```python
from build123d import *

# Parameters (mm, degrees)
EXTRUDE_448_DEPTH     = 2
SKETCH_2_R            = 2
CUT_EXTRUDE_659_DEPTH = 83.412799184
SKETCH_3_R            = 2
CUT_EXTRUDE_885_DEPTH = 83.412799184


with BuildPart() as part:
    # Эскиз1 → Extrude 448 (new body)
    with BuildSketch(Plane(origin=(0, 0, 0), x_dir=(1, 0, 0), z_dir=(0, 1, 0))):
        with BuildLine():
            Line((-77.703225806, 4.495408688), (-0.361290323, 7.991837667))
            Line((-0.361290323, 7.991837667), (0.361290323, 7.991837667))
            Line((0.361290323, 7.991837667), (77.703225806, 4.495408688))
            ThreePointArc((77.703225806, 4.495408688), (82, 0), (77.703225806, -4.495408688))
            Line((77.703225806, -4.495408688), (0.361290323, -7.991837667))
            Line((0.361290323, -7.991837667), (-0.361290323, -7.991837667))
            Line((-0.361290323, -7.991837667), (-77.703225806, -4.495408688))
            ThreePointArc((-77.703225806, -4.495408688), (-82, 0), (-77.703225806, 4.495408688))
        make_face()
    extrude(amount=EXTRUDE_448_DEPTH)

    # Эскиз2 → Cut-Extrude 659 (cut, through all)
    with BuildSketch(Plane(origin=(0, 2, 0), x_dir=(1, 0, 0), z_dir=(0, 1, 0))):
        with Locations(Location((0, 0, 0), (0, 0, 270))):
            Circle(SKETCH_2_R)
    extrude(amount=-CUT_EXTRUDE_659_DEPTH, mode=Mode.SUBTRACT)

    # Эскиз3 → Cut-Extrude 885 (cut, through all)
    with BuildSketch(Plane(origin=(0, 2, 0), x_dir=(1, 0, 0), z_dir=(0, 1, 0))):
        with Locations(Location((-77.5, 0, 0), (0, 0, 270))):
            Circle(SKETCH_3_R)
        with Locations(Location((77.5, 0, 0), (0, 0, 270))):
            Circle(SKETCH_3_R)
    extrude(amount=-CUT_EXTRUDE_885_DEPTH, mode=Mode.SUBTRACT)


solid = part.part
```
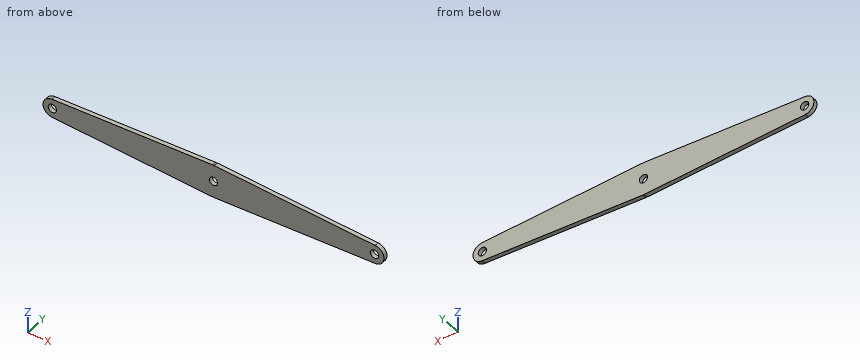
CAD build for the part. Positions are in the model's coordinates, mm. Round coordinates to 2 decimals unless told otherwise and drop trailing zeros. Write each loop counter-clockwise with the first axis right and the second up, starting at its lowest first coordinate (ties: lowest second). Pieces come first, ordered by that corner, then holes. Notation, with made-up numbers: (-18.75, -3.75) - (26.25, -3.75) arc R29 cw to (26.25, 27.25) - close; hole circle Ø4 at (77.5, 44). An arc over 180 degrees is marked (long way). Write item = value, one per line. Start each with the question number.
Q1. Band-saw the part on C-C (x = -35.5). Give the cut face in (y, z), then the cut area to 3 significant figures.
Q2. Band-saw the part on B-B (y = 1.15). Give the cut face in (x, z), then the cut area to 3 significant figures.
Q3. Band-saw the part on A-A (z = 0). Give the cut face in (x, y).
Q4. Drop a flat-ended pin along its axis: pin 1 (1.5 mm diameter, centred on x = -58.5, z = 6.5, fed in from -Y). Give the stop position or say it passes through.
Q5. Band-saw the part on D-D (x = 20.5). Give the cut face in (y, z).
Q6. Probe L1, parallel to Z at x = 37, y = 1.4; L2, parallel to Z at x = 66.5, y = 0.65. List the from-to ranges inside material, lowest first. Write a range as from..to.
Answers below:
q1.outline = (0, -6.4) - (2, -6.4) - (2, 6.4) - (0, 6.4) - close
q1.area = 25.6 mm2
q2.outline = (-77.7, -4.5) - (-0.36, -7.99) - (0.36, -7.99) - (77.7, -4.5) arc R4.5 ccw to (77.7, 4.5) - (0.36, 7.99) - (-0.36, 7.99) - (-77.7, 4.5) arc R4.5 ccw to start; hole circle Ø4 at (-77.5, 0); hole circle Ø4 at (0, 0); hole circle Ø4 at (77.5, 0)
q2.area = 1,970 mm2
q3.outline = (-82, 0) - (-79.5, 0) - (-79.5, 2) - (-82, 2) - close; (-75.5, 0) - (-2, 0) - (-2, 2) - (-75.5, 2) - close; (2, 0) - (75.5, 0) - (75.5, 2) - (2, 2) - close; (79.5, 0) - (82, 0) - (82, 2) - (79.5, 2) - close
q4.pin_1 = through
q5.outline = (0, -7.08) - (2, -7.08) - (2, 7.08) - (0, 7.08) - close
q6.L1 = -6.34..6.34
q6.L2 = -5..5
